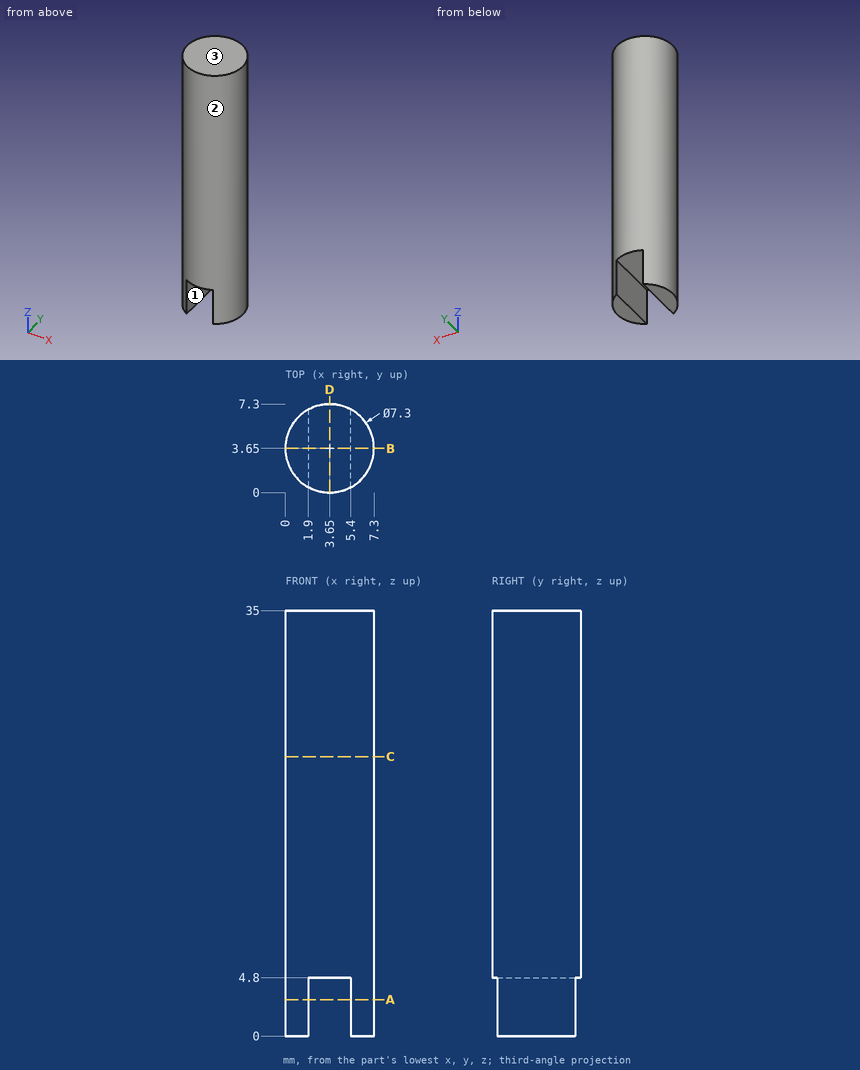
For this review, use the dimensioned drawing (mm, ordinates from the lowest corner) and the shaded views. Round coordinates to 2 decimals unless told otherwise and drop trailing zeros. Order: outer loops, then holes, each group sorted by start corner. A loop starts at its lowest first (then second) coordinate and runs counter-clockwise, first axis right, second up. Notation, with made-up numbers: (35.5, 67) -> (82.5, 67) arc R17 cw to (82.5, 84) -> close; hole circle Ø8 at (28, 73.5). An arc over 180 degrees is marked (long way). Use CSV: the item, a comma, the result in double quotes. Start each with the question number.
(1) Insertion check: pin 1 (1.5 mm diameter, centred on x = 5.5, z = 28, fed in from +Y). The pin has a flat end and moves straight along its axis. Give the tip position at first contact, or say it passes through.
(2) Wall thickness on probe 1 along Z at (x, y) = (3.5, 5.75); probe 2 along X at (y, z) = (4.25, 2); probe 3 along Y at (x, z) = (2, 19): over which ranges is each line inside the solid? List them lowest first. Write a range as from..to.
(3) Consider section B-B on y = 3.65. Write out the cut boundary in (x, z), and give its area (3 significant figures).
(4) Consider section C-C on z = 23. Write out the cut boundary in (x, y), and give its area (3 significant figures).
(5) Mouldability with a two-part tool opening along X and no side actions: class the marked faces 1, 2 and 3 as pulls with the +X half, pulls with the -X half, needs draft (parallel to the pull), parting line crosses it, or undercut.
(6) Consider section A-A on z = 3. Write out the cut boundary in (x, y), and give its area (3 significant figures).
(7) Consider section D-D on x = 3.65. Write out the cut boundary in (y, z), and give its area (3 significant figures).
Responses:
1,pin 1,"y = 7.13"
2,probe 1,"4.8..35"
2,probe 2,"0.05..1.9, 5.4..7.25"
2,probe 3,"0.39..6.91"
3,outline,"(0, 0) -> (1.9, 0) -> (1.9, 4.8) -> (5.4, 4.8) -> (5.4, 0) -> (7.3, 0) -> (7.3, 35) -> (0, 35) -> close"
3,area,"239 mm²"
4,outline,"circle Ø7.3 at (3.65, 3.65)"
4,area,"41.9 mm²"
5,face 1,"undercut"
5,face 2,"parting line crosses it"
5,face 3,"needs draft"
6,outline,"(1.9, 0.45) -> (1.9, 6.85) arc R3.65 ccw to start; (5.4, 0.45) arc R3.65 ccw to (5.4, 6.85) -> close"
6,area,"17.3 mm²"
7,outline,"(0, 4.8) -> (7.3, 4.8) -> (7.3, 35) -> (0, 35) -> close"
7,area,"220 mm²"
